Autodesk Inventor part; units mm, degrees
ref_plane "YZ Plane" through (0, 0, 0) normal (1, 0, 0) x (0, 1, 0)
ref_plane "XZ Plane" through (0, 0, 0) normal (0, 1, 0) x (-1, 0, 0)
ref_plane "XY Plane" through (0, 0, 0) normal (0, 0, 1) x (1, 0, 0)
sketch "Sketch1" plane through (0, 0, 0) normal (1, 0, 0) x (0, 1, 0)
  line L0 (0, 0) -> (1.5875, 0)
  line L1 (1.5875, 0) -> (1.5875, -50.8)
  line L2 (1.5875, -50.8) -> (0, -50.8)
  line L3 (0, -50.8) -> (0, 0)
  line L4 (1.5875, 0) -> (45.5816, -25.4)
  line L5 (45.5816, -25.4) -> (44.7878, -26.7748)
  line L6 (44.7878, -26.7748) -> (0.7938, -1.3748)
  line L7 (0.7938, -1.3748) -> (1.5875, 0)
  line L8 (1.5875, 0) -> (52.3875, 0) construction
  dimension "d0" = 1.5875
  dimension "d1" = 50.8
  dimension "d2" = 50.8
  dimension "d3" = 30
  dimension "d4" = 1.5875
extrude "Extrusion1" add sketch "Sketch1" along normal blind 304.8
sketch "Sketch2" plane through (0, 0, -50.8) normal (0, -1, 0) x (1, 0, 0)
  line L0 (0, 0) -> (304.8, 0)
  line L1 (304.8, 50.8) -> (304.8, 0)
  point P0 (177.8, 28.575)
  point P1 (127, 28.575)
  dimension "d7" = 28.575
  dimension "d8" = 28.575
  dimension "d9" = 127
  dimension "d10" = 177.8
hole "Hole1" at (177.8, 0, -22.225) at (127, 0, -22.225) direction (0, 1, 0) diameter 6.35 depth 6.35 tip angle 118
sketch "Sketch5" plane through (0, 1.5875, -1.8331) normal (0, 1, 0) x (1, 0, 0)
  line L0 (0, 48.9669) -> (304.8, 48.9669)
  line L1 (0, 48.9669) -> (101.6, 48.9669)
  line L2 (101.6, 48.9669) -> (101.6, 23.5669)
  line L3 (101.6, 23.5669) -> (0, 23.5669)
  line L4 (0, 23.5669) -> (0, 48.9669)
  line L5 (304.8, 48.9669) -> (203.2, 48.9669)
  line L6 (203.2, 48.9669) -> (203.2, 23.5669)
  line L7 (203.2, 23.5669) -> (304.8, 23.5669)
  line L8 (304.8, 23.5669) -> (304.8, 48.9669)
  line L9 (203.2, 48.9669) -> (177.8, 48.9669)
  line L10 (177.8, 48.9669) -> (203.2, 23.5669)
  line L11 (101.6, 48.9669) -> (127, 48.9669)
  line L12 (0, 48.9669) -> (304.8, 48.9669)
  line L13 (127, 48.9669) -> (101.6, 23.5669)
  point P0 (0, -1.8331)
  dimension "d28" = 101.6
  dimension "d29" = 25.4
  dimension "d30" = 101.6
  dimension "d31" = 25.4
  dimension "d32" = 25.4
  dimension "d33" = 25.4
extrude "Extrusion4" cut sketch "Sketch5" against normal blind 6.35
properties part number "stopper plate" material "Aluminum 6061"
For this review, take the finished solid that the model builds, in its own axes (mm). A direction names the side the tool comes from. Coordinates: 2 decimals unless noted, no trailing zeros. Loops run counter-clockwise (first coordinate to the right, second up) from the corner with the lowest first, then second, coordinate; pieces in that order, holes last. Notation, with made-up numbers: (11.25, -35) -> (44.25, -35) arc R20 cw to (44.25, -28) -> close; hole circle Ø5 at (75.5, 62.5). An arc over 180 degrees is marked (long way). Return JSON: item names as keys, results as strings. Group by question number.
(1) Tool access review of faces 4 (the cylindrical face through (174.652, 0.805, -21.812)), 5 (the flat face through (150, 0, -20)), 6 (the flat face through (150, 1.588, -21)): name each direction out of +Z, -Z, +X, -X, +Y, -Y from which nothing blocks a thin tool from reaching the whole face with its end or side.
(2) Consider section A-A, the plane x = 82. Give the boundary of the cut face in (y, z), plus the area to 3 significant figures.
(3) For pin 1 Ø3 at (x, y) = (115.5, 37) entering from -Z; pin 2 Ø1.7 at (x, y) = (279, 1) entering from -Z; pin 3 Ø1 at (x, y) = (198, 37) entering from +Z; pin 4 Ø8 at (y, z) = (7.5, -17.5) entering from +X, all flat-tipped, find the tip position at first contact; note any pin that passes through.
(4) To check wall thickness, follow L1, parallel to Z at x = 177.8, y = 1; L2, parallel to Y at x = 188, z = -29.5; L3, parallel to Y at x = 31.5, z = -23. State the ranges of each line that lie inside material, in increasing order.
(5) Consider section D-D, the plane z = -31. Give the boundary of the cut face in (x, y), plus the area to 3 significant figures.
(6) Consider section B-B, the plane z = -8. Give the boundary of the cut face in (x, y).
(7) Mouldability with a two-part tool opening along Z and no side actions: class faces 1 (the cylindrical face through (123.852, 0.805, -21.812)), 2 (the flat face through (304.8, 18, -10)), 3 (the flat face through (114.5, 0.8, -38.3)) as pulls with the +Z half, pulls with the -Z half, needs draft (parallel to the pull), parting line crosses it, or undercut.
(8) Consider section C-C, the plane x = 155. Give the boundary of the cut face in (y, z), plus the area to 3 significant figures.
Results below:
{
 "1": {"face 4": "-Y", "face 5": "+Z, -Z, +X, -X, -Y", "face 6": "-Z, +X, -X"},
 "2": {"outline": "(0, -25.4) -> (1.59, -25.4) -> (1.59, -1.83) -> (44.79, -26.77) -> (45.58, -25.4) -> (1.59, 0) -> (0, 0) -> close", "area": "120 mm2"},
 "3": {"pin 1": "stops at z = -23.14", "pin 2": "stops at z = -25.4", "pin 3": "stops at z = -20.16", "pin 4": "passes through"},
 "4": {"L1": "z = -50.8 to -25.4, -19.05 to 0", "L2": "y = 0 to 1.59", "L3": "y = 0 to 1.59, 38.25 to 41.42"},
 "5": {"outline": "(107.2, 0) -> (197.6, 0) -> (197.6, 1.59) -> (107.2, 1.59) -> close", "area": "144 mm2"},
 "6": {"outline": "(0, 0) -> (304.8, 0) -> (304.8, 1.59) -> (0, 1.59) -> close; (0, 12.27) -> (304.8, 12.27) -> (304.8, 15.44) -> (0, 15.44) -> close"},
 "7": {"face 1": "undercut", "face 2": "needs draft", "face 3": "pulls with the -Z half"},
 "8": {"outline": "(0, -50.8) -> (1.59, -50.8) -> (1.59, -1.83) -> (44.79, -26.77) -> (45.58, -25.4) -> (1.59, 0) -> (0, 0) -> close", "area": "161 mm2"}
}
